```python
from build123d import *

# Parameters (mm, degrees)
SKETCH_1_R      = 1.625
SKETCH_1_R_2    = 1.575
EXTRUDE_1_DEPTH = 5
CHAMFER_1_SIZE  = 0.5
EXTRUDE_2_DEPTH = 5
EXTRUDE_3_DEPTH = 5


with BuildPart() as part:
    # 草图1 → 凸台-拉伸1 (new body)
    with BuildSketch(Plane(origin=(-2.5, 0, 0), x_dir=(0, -1, 0), z_dir=(-1, 0, 0))):
        with BuildLine():
            Line((-13.615329727, 4.634814191), (-5.764611689, -4.797838271))
            ThreePointArc((-5.764611689, -4.797838271), (4.504097017, -5.996925051), (6.214285714, 4.199125273))
            ThreePointArc((6.214285714, 4.199125273), (4.938171125, 6.870258752), (4.5, 9.797958971))
            Line((4.5, 9.797958971), (4.5, 90.687804581))
            ThreePointArc((4.5, 90.687804581), (4.50486974, 90.999847969), (4.519474215, 91.311587443))
            Line((4.519474215, 91.311587443), (5.970120756, 114.521932102))
            ThreePointArc((5.970120756, 114.521932102), (6.011395859, 114.998738119), (6.075436578, 115.473023263))
            Line((6.075436578, 115.473023263), (7.406407472, 123.818844483))
            ThreePointArc((7.406407472, 123.818844483), (1.981957648, 132.233383985), (-6.974045822, 127.759109434))
            Line((-6.974045822, 127.759109434), (-13.335850238, 111.678734019))
            ThreePointArc((-13.335850238, 111.678734019), (-13.841506721, 109.968181983), (-14.03521939, 108.195006258))
            Line((-14.03521939, 108.195006258), (-15.927277723, 11.227016703))
            ThreePointArc((-15.927277723, 11.227016703), (-15.365674922, 7.722463826), (-13.615329727, 4.634814191))
        make_face()
        with Locations(Location((0, 125, 0), (0, 0, 270))):
            Circle(SKETCH_1_R, mode=Mode.SUBTRACT)
        with Locations(Location((-8.5, 23.5, 0), (0, 0, 270))):
            Circle(SKETCH_1_R_2, mode=Mode.SUBTRACT)
        with Locations(Location((-5, 106.5, 0), (0, 0, 270))):
            Circle(SKETCH_1_R_2, mode=Mode.SUBTRACT)
        with Locations(Location((0, 0, 0), (0, 0, 270))):
            Circle(SKETCH_1_R, mode=Mode.SUBTRACT)
        with BuildLine():
            Line((-8.259933132, 32.545201991), (-6.991881816, 97.532831936))
            ThreePointArc((-6.991881816, 97.532831936), (-4.95324547, 99.493434355), (-2.992643051, 97.454798009))
            Line((-2.992643051, 97.454798009), (-4.260694367, 32.467168064))
            ThreePointArc((-4.260694367, 32.467168064), (-6.299330713, 30.506565645), (-8.259933132, 32.545201991))
        make_face(mode=Mode.SUBTRACT)
    extrude(amount=-EXTRUDE_1_DEPTH)

    # 倒角1
    chamfer_1_edges = [part.edges().sort_by_distance(p)[0] for p in [
        (2.5, -4.504097017, -5.996925051),
        (-2.5, 14.981248556, 59.71101148),
        (-2.5, 13.841506721, 109.968181983),
        (-2.5, 10.15494803, 119.718921727),
        (-2.5, -1.981957648, 132.233383985),
        (-2.5, -6.740922025, 119.645933873),
        (-2.5, -6.011395859, 114.998738119),
        (-2.5, -5.244797486, 102.916759772),
        (-2.5, -4.50486974, 90.999847969),
        (-2.5, -4.5, 50.242881776),
        (-2.5, -4.938171125, 6.870258752),
        (2.5, -4.938171125, 6.870258752),
        (-2.5, -4.504097017, -5.996925051),
        (-2.5, 9.689970708, -0.08151204),
        (-2.5, 15.365674922, 7.722463826),
        (2.5, -4.5, 50.242881776),
        (2.5, -4.50486974, 90.999847969),
        (2.5, -5.244797486, 102.916759772),
        (2.5, -6.011395859, 114.998738119),
        (2.5, 0, 126.625),
        (-2.5, 0, 126.625),
        (2.5, -6.740922025, 119.645933873),
        (2.5, 8.5, 25.075),
        (-2.5, 8.5, 25.075),
        (2.5, -1.981957648, 132.233383985),
        (2.5, 6.299330713, 30.506565645),
        (2.5, 7.625907474, 65.039016964),
        (2.5, 4.95324547, 99.493434355),
        (2.5, 3.626668709, 64.960983036),
        (2.5, 10.15494803, 119.718921727),
        (-2.5, 6.299330713, 30.506565645),
        (-2.5, 3.626668709, 64.960983036),
        (-2.5, 4.95324547, 99.493434355),
        (-2.5, 7.625907474, 65.039016964),
        (2.5, 13.841506721, 109.968181983),
        (2.5, 15.365674922, 7.722463826),
        (2.5, 14.981248556, 59.71101148),
        (2.5, 5, 108.075),
        (-2.5, 5, 108.075),
        (2.5, 0, 1.625),
        (-2.5, 0, 1.625),
        (2.5, 9.689970708, -0.08151204),
    ]]
    chamfer(chamfer_1_edges, length=CHAMFER_1_SIZE)

    # Sketch 3D_1 → 凸台-拉伸2 (add)
    with BuildSketch(Plane(origin=(2.5, -0.12857826, 115.032359126), x_dir=(0, -0.013604097539647628, -0.9999074599832386), z_dir=(1, 0, 0))):
        Polygon((0, 0), (96.922582011, 1.318666289), (96.940522936, 0), (0.017940925, -1.318666289), align=None)
    extrude(amount=-EXTRUDE_2_DEPTH)

    # Sketch 3D_2 → 凸台-拉伸3 (add)
    with BuildSketch(Plane(origin=(2.5, 7.131907218, 114.778535538), x_dir=(0, -0.036322969616865465, -0.9993401032072177), z_dir=(1, 0, 0))):
        Polygon((0, 0), (17.760330703, 3.73858914), (75.88295175, 7.788553229), (95.2811606, 9.140213698), (100.246342151, 0), (71.295283996, -6.76874803), (5.48633166, -7.137591509), align=None)
    extrude(amount=-EXTRUDE_3_DEPTH)


solid = part.part
```
Could you check a few things on this model? Use its own coordinates, in mm. A direction names the side the tool comes from. Give positions to 0.01 mm unless a question says otherwise; leave off trailing zeros. Order: outer loops, then holes, each group sorted by start corner. A loop starts at its lowest first (then second) coordinate and runs counter-clockwise, first axis right, second up.
Q1. If I drill on line 1 along Z through (x, y) = (-1.25, 1); line 2 along Z through (x, y) = (-2.3, -0.5); line 3 along Y through (x, z) = (-0.8, 0) (3 decimals), over which ranges is the centre line in solid material (lowest first)?
Q2. Suppose I cut it at B-B, the plane x = 0.6. Write out the boundary of the cut face in (y, z) (3 decimals).
Q3. For faces 1 (the cylindrical face through (-0.03, -4.38, -6.09)), 2 (the flat face through (-0.03, -6.73, 119.59)), which set-ups out of +Z, -Z, +X, -X, +Y, -Y let a thin tool reach every point of the face, with its end or its side?
Q4. Suppose I cut it at A-A, the plane y = 0. Write out the boundary of the cut face in (x, z) (3 decimals).
Q5. We'd pull the mould along Y, two halves only. Please class faces 3 (the cylindrical face through (-0.028, -0.071, 126.623)), 4 (the flat face through (-2.5, 4, 63)), 5 (the flat face through (2.254, 9.55, 0.147)), 6 (the cylindrical face through (-0.03, -4.95, 6.83)): +Y half, -Y half, draft (parallel to the pull), parting line (faces both ways), or undercut.
Q6. I'm going to push flat-ended pins straight in: P1, Ø3, axis at x = 0, y = 5, coming from the +Z side; P2, Ø2, axis at x = 0, z = 111, coming from the -Y side; P3, Ø1.2, axis at x = 1, z = 33, coming from the -Y side; P4, Ø1.9, axis at y = 0, z = 125, coming from the +X side. Where does each tip first touch, or does it pass through?
Q7. Suppose I cut it at C-C, the plane z = 66.5. Write out the boundary of the cut face in (x, y), and give its area (3 significant figures).
Solution:
1. line 1: z = -7.43 to -1.28, 1.28 to 123.72, 126.28 to 132.43
1. line 2: z = -7.18 to -1.86, 1.86 to 123.14, 126.86 to 132.18
1. line 3: y = -7.5 to -1.625, 1.625 to 9.758
2. outline: (-7.406, 123.819) - (-6.075, 115.473) arc R10 cw to (-5.97, 114.522) - (-4.519, 91.312) arc R10 cw to (-4.5, 90.688) - (-4.5, 9.798) arc R10 cw to (-6.214, 4.199) arc R7.5 ccw to (5.765, -4.798) - (13.615, 4.635) arc R10 ccw to (15.927, 11.227) - (14.035, 108.195) arc R10 ccw to (13.336, 111.679) - (6.974, 127.759) arc R7.5 ccw to start; hole circle Ø3.25 at (0, 0); hole circle Ø3.25 at (0, 125)
3. face 1: +X, -X
3. face 2: +X, -X, -Y
4. outline: (-2.5, -7) - (-2, -7.5) - (2, -7.5) - (2.5, -7) - (2.5, -2.125) - (2, -1.625) - (-2, -1.625) - (-2.5, -2.125) - close; (-2.5, 2.125) - (-2, 1.625) - (2, 1.625) - (2.5, 2.125) - (2.5, 122.875) - (2, 123.375) - (-2, 123.375) - (-2.5, 122.875) - close; (-2.5, 127.125) - (-2, 126.625) - (2, 126.625) - (2.5, 127.125) - (2.5, 132) - (2, 132.5) - (-2, 132.5) - (-2.5, 132) - close
5. face 3: undercut
5. face 4: draft
5. face 5: +Y half
5. face 6: -Y half
6. P1: stops at z = 131.63
6. P2: stops at y = -5.81
6. P3: stops at y = -4.5
6. P4: passes through
7. outline: (-2.5, -4) - (-2, -4.5) - (2, -4.5) - (2.5, -4) - (2.5, 14.35) - (2, 14.85) - (-2, 14.85) - (-2.5, 14.35) - close
7. area: 96.2 mm2
